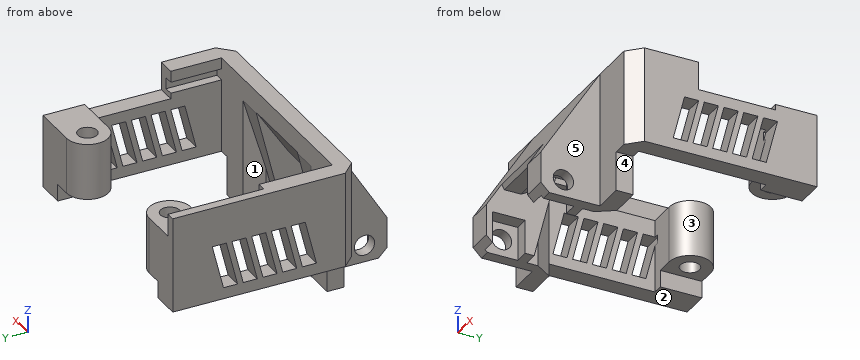
from build123d import *

# Parameters (mm, degrees)
SKETCH_1_W           = 44
SKETCH_1_H           = 34
EXTRUDE_1_DEPTH      = 24
CUT_EXTRUDE_1_DEPTH  = 31
SKETCH_5_W           = 23
SKETCH_5_H           = 10.5
EXTRUDE_4_DEPTH      = 1
EXTRUDE_5_DEPTH      = 23
SKETCH_7_R           = 1.8
CUT_EXTRUDE_2_DEPTH  = 23
CUT_EXTRUDE_4_DEPTH  = 19
CHAMFER_2_SIZE       = 2
CHAMFER_2_SIZE2      = 3
SKETCH_11_R          = 1.7
EXTRUDE_6_DEPTH      = 20
CUT_EXTRUDE_7_DEPTH  = 4
CHAMFER_3_SIZE       = 2.4
SKETCH_14_W          = 40.8
SKETCH_14_H          = 4
CUT_EXTRUDE_8_DEPTH  = 18
SKETCH_15_W          = 44
SKETCH_15_H          = 1
CUT_EXTRUDE_9_DEPTH  = 24
SKETCH_16_W          = 3.2
SKETCH_16_H          = 13.6
CUT_EXTRUDE_10_DEPTH = 5
SKETCH_17_W          = 1.6
SKETCH_17_H          = 4
CUT_EXTRUDE_11_DEPTH = 7.4
CUT_EXTRUDE_12_DEPTH = 7
SKETCH_19_W          = 1
SKETCH_19_H          = 10.5
CUT_EXTRUDE_13_DEPTH = 23
CHAMFER_4_SIZE       = 1.5
CHAMFER_5_SIZE       = 3
CHAMFER_5_SIZE2      = 2
CUT_EXTRUDE_START    = -3
SKETCH_20_W          = 14
SKETCH_20_H          = 11.956557484
CUT_EXTRUDE_14_DEPTH = 17
CHAMFER_6_SIZE       = 10
CHAMFER_6_SIZE_2     = 4
CHAMFER_7_SIZE       = 1
SKETCH_22_W          = 6.7
SKETCH_22_H          = 10
CUT_EXTRUDE_15_DEPTH = 10
SKETCH_24_W          = 6
SKETCH_24_H          = 5.8
CUT_EXTRUDE_16_DEPTH = 2.5


with BuildPart() as part:
    # Sketch 1 → Extrude 1 (new body)
    with BuildSketch(Plane.XY):
        with Locations((0, 27)):
            Rectangle(SKETCH_1_W, SKETCH_1_H)
    extrude(amount=EXTRUDE_1_DEPTH)

    # Sketch 2 → Cut-Extrude 1 (cut)
    with BuildSketch(Plane(origin=(0, 44, 0), x_dir=(1, 0, 0), z_dir=(0, 1, 0))):
        Polygon((-18.8, 0), (18.8, 0), (18.8, -20), (20.4, -20), (20.4, -22), (18.8, -22), (18.8, -24), (-18.8, -24), (-18.8, -22), (-20.4, -22), (-20.4, -20), (-18.8, -20), align=None)
    extrude(amount=-CUT_EXTRUDE_1_DEPTH, mode=Mode.SUBTRACT)



with BuildPart() as body_2:
    # Sketch 5 → Extrude 4 (new body)
    with BuildSketch(Plane(origin=(0, 0, 0), x_dir=(-1, 0, 0), z_dir=(0, 0, -1))):
        with Locations((0, 4.75)):
            Rectangle(SKETCH_5_W, SKETCH_5_H)
    extrude(amount=EXTRUDE_4_DEPTH)


with BuildPart() as part_1:
    add(part.part)

    add(body_2.part)  # Extrude 5 merges body 2
    # Sketch 6 → Extrude 5 (add)
    with BuildSketch(Plane(origin=(11.5, 0, 0), x_dir=(0, 0, -1), z_dir=(1, 0, 0))):
        Polygon((0, -0.5), (-7, -0.5), (-24, 10), (0, 10), align=None)
    extrude(amount=-EXTRUDE_5_DEPTH)

    # Sketch 7 → Cut-Extrude 2 (cut)
    with BuildSketch(Plane.ZY.offset(11.5)):
        with Locations(Location((3, 3.5, 0), (0, 0, 270))):
            Circle(SKETCH_7_R)
    extrude(amount=-CUT_EXTRUDE_2_DEPTH, mode=Mode.SUBTRACT)

    # Sketch 8 → Cut-Extrude 4 (cut)
    with BuildSketch(Plane.ZY.offset(9.5)):
        Polygon((0, 8), (20, 13), (0, 13), align=None)
    extrude(amount=-CUT_EXTRUDE_4_DEPTH, mode=Mode.SUBTRACT)

    # Chamfer 2
    chamfer_2_edges = [part_1.edges().sort_by_distance(p)[0] for p in [
        (9.5, 13, 10),
    ]]
    chamfer_2_side = [part_1.faces().sort_by_distance(p)[0] for p in [
        (-18.32664601, 13, 10),
    ]]
    chamfer(chamfer_2_edges, length=CHAMFER_2_SIZE, length2=CHAMFER_2_SIZE2, reference=chamfer_2_side[0])

    # Sketch 11 → Extrude 6 (add)
    # profile 1 of 2: a face of its own
    with BuildSketch(Plane(origin=(0, 0, 0), x_dir=(-1, 0, 0), z_dir=(0, 0, -1))):
        with BuildLine():
            Line((-14, 43), (-18.8, 43))
            Line((-18.8, 43), (-18.8, 35.6))
            Line((-18.8, 35.6), (-14, 35.6))
            ThreePointArc((-14, 35.6), (-10.3, 39.3), (-14, 43))
        make_face()
        with Locations((-14, 39.3)):
            Circle(SKETCH_11_R, mode=Mode.SUBTRACT)
    # profile 2 of 2: a face of its own
    with BuildSketch(Plane(origin=(0, 0, 0), x_dir=(-1, 0, 0), z_dir=(0, 0, -1))):
        with BuildLine():
            Line((18.8, 35.6), (14, 35.6))
            ThreePointArc((14, 35.6), (10.3, 39.3), (14, 43))
            Line((14, 43), (18.8, 43))
            Line((18.8, 43), (18.8, 35.6))
        make_face()
        with Locations((14, 39.3)):
            Circle(SKETCH_11_R, mode=Mode.SUBTRACT)
    extrude(amount=-EXTRUDE_6_DEPTH)

    # Sketch 13 → Cut-Extrude 7 (cut)
    with BuildSketch(Plane.ZY.offset(22)):
        Polygon((9, 34), (17, 36), (17, 33.5), (9, 31.5), align=None)
        Polygon((9, 30.5), (17, 32.5), (17, 30), (9, 28), align=None)
        Polygon((9, 27), (17, 29), (17, 26.5), (9, 24.5), align=None)
        Polygon((9, 23.5), (17, 25.5), (17, 23), (9, 21), align=None)
        Polygon((9, 20), (17, 22), (17, 19.5), (9, 17.5), align=None)
    cut_extrude_7 = extrude(amount=-CUT_EXTRUDE_7_DEPTH, mode=Mode.SUBTRACT)

    # Mirror 1: Cut-Extrude 7 across plane
    add(cut_extrude_7.mirror(Plane(origin=(0, 0, 0), x_dir=(0, 0, 1), z_dir=(1, 0, 0))), mode=Mode.SUBTRACT)

    # Chamfer 3
    chamfer_3_edges = [part_1.edges().sort_by_distance(p)[0] for p in [
        (22, 10, 12),
        (-22, 10, 12),
    ]]
    chamfer(chamfer_3_edges, length=CHAMFER_3_SIZE)

    # Sketch 14 → Cut-Extrude 8 (cut)
    with BuildSketch(Plane(origin=(0, 44, 0), x_dir=(1, 0, 0), z_dir=(0, 1, 0))):
        with Locations((0, -22)):
            Rectangle(SKETCH_14_W, SKETCH_14_H)
    extrude(amount=-CUT_EXTRUDE_8_DEPTH, mode=Mode.SUBTRACT)

    # Sketch 15 → Cut-Extrude 9 (cut)
    with BuildSketch(Plane(origin=(0, 0, 0), x_dir=(-1, 0, 0), z_dir=(0, 0, -1))):
        with Locations((0, 43.5)):
            Rectangle(SKETCH_15_W, SKETCH_15_H)
    extrude(amount=-CUT_EXTRUDE_9_DEPTH, mode=Mode.SUBTRACT)

    # Sketch 16 → Cut-Extrude 10 (cut)
    with BuildSketch(Plane.XY.offset(24)):
        with Locations((20.4, 28.8)):
            Rectangle(SKETCH_16_W, SKETCH_16_H)
    extrude(amount=-CUT_EXTRUDE_10_DEPTH, mode=Mode.SUBTRACT)

    # Sketch 17 → Cut-Extrude 11 (cut)
    with BuildSketch(Plane(origin=(0, 43, 0), x_dir=(1, 0, 0), z_dir=(0, 1, 0))):
        with Locations((21.2, -22)):
            Rectangle(SKETCH_17_W, SKETCH_17_H)
    extrude(amount=-CUT_EXTRUDE_11_DEPTH, mode=Mode.SUBTRACT)

    # Sketch 18 → Cut-Extrude 12 (cut)
    with BuildSketch(Plane(origin=(0, 0, 0), x_dir=(-1, 0, 0), z_dir=(0, 0, -1))):
        Polygon((-22, 43), (-17, 43), (-17, 10), (-19.6, 10), (-22, 12.4), align=None)
        Polygon((22, 12.4), (19.6, 10), (17, 10), (17, 43), (22, 43), align=None)
    extrude(amount=-CUT_EXTRUDE_12_DEPTH, mode=Mode.SUBTRACT)

    # Sketch 19 → Cut-Extrude 13 (cut)
    with BuildSketch(Plane.ZY.offset(11.5)):
        with Locations((-0.5, 4.75)):
            Rectangle(SKETCH_19_W, SKETCH_19_H)
    extrude(amount=-CUT_EXTRUDE_13_DEPTH, mode=Mode.SUBTRACT)

    # Chamfer 4
    chamfer_4_edges = [part_1.edges().sort_by_distance(p)[0] for p in [
        (0, -0.5, 0),
    ]]
    chamfer(chamfer_4_edges, length=CHAMFER_4_SIZE)

    # Chamfer 5
    chamfer_5_edges = [part_1.edges().sort_by_distance(p)[0] for p in [
        (-9.5, 13, 10),
    ]]
    chamfer_5_side = [part_1.faces().sort_by_distance(p)[0] for p in [
        (-9.5, 11.333333333, 6.666666667),
    ]]
    chamfer(chamfer_5_edges, length=CHAMFER_5_SIZE, length2=CHAMFER_5_SIZE2, reference=chamfer_5_side[0])

    # Sketch 20 → Cut-Extrude 14 (cut)
    with BuildSketch(Plane(origin=(0, 0, 0), x_dir=(1, 0, 0), z_dir=(0, 1, 0)).offset(CUT_EXTRUDE_START)):
        with Locations((0, -4.591721258)):
            Rectangle(SKETCH_20_W, SKETCH_20_H)
    extrude(amount=CUT_EXTRUDE_14_DEPTH, mode=Mode.SUBTRACT)

    # Chamfer 6
    # the kernel refuses this chamfer: 10, 4 mm, written as the material it takes off along each edge
    with BuildSketch(Plane(origin=(7, 10.6425, 10.57), x_dir=(0, 0.254985552304956, 0.966944863017399), z_dir=(-1, 0, 0))) as chamfer_6_piece_1:
        Polygon((CHAMFER_6_SIZE * 0.999917387214, -CHAMFER_6_SIZE * 0.0128537444865), (-CHAMFER_6_SIZE_2 * 0.254985552305, -CHAMFER_6_SIZE_2 * 0.966944863017), (0, 0), align=None)
    extrude(amount=14, mode=Mode.SUBTRACT)

    # Chamfer 7
    chamfer_7_edges = [part_1.edges().sort_by_distance(p)[0] for p in [
        (0, 1.705, 10.57),
        (0, 6.6425, 10.57),
    ]]
    chamfer(chamfer_7_edges, length=CHAMFER_7_SIZE)

    # Sketch 22 → Cut-Extrude 15 (cut)
    with BuildSketch(Plane(origin=(0, 43, 0), x_dir=(1, 0, 0), z_dir=(0, 1, 0))):
        with Locations((13.65, -5)):
            Rectangle(SKETCH_22_W, SKETCH_22_H)
        with Locations((-13.65, -5)):
            Rectangle(SKETCH_22_W, SKETCH_22_H)
    extrude(amount=-CUT_EXTRUDE_15_DEPTH, mode=Mode.SUBTRACT)

    # Sketch 24 → Cut-Extrude 16 (cut)
    with BuildSketch(Plane(origin=(-7, 0, 0), x_dir=(0, 0, -1), z_dir=(1, 0, 0))):
        with Locations((-3, 3.5)):
            Rectangle(SKETCH_24_W, SKETCH_24_H)
    cut_extrude_16 = extrude(amount=-CUT_EXTRUDE_16_DEPTH, mode=Mode.SUBTRACT)

    # Mirror 2: Cut-Extrude 16 across plane
    add(cut_extrude_16.mirror(Plane(origin=(0, 0, 0), x_dir=(0, 0, 1), z_dir=(1, 0, 0))), mode=Mode.SUBTRACT)


solid = part_1.part
Design review of the part built by this model. Coordinates are the model's own, in mm. Face numbers are marked on the shaded views. A direction names the side the tool comes from. Give positions to 0.01 mm unless a question says otherwise; leave off trailing zeros. Write each loop counter-clockwise with the first axis right and the second up, starting at its lowest first coordinate (ties: lowest second). Pieces come first, ordered by that corner, then holes. Notation, with made-up numbers: M 62,61 L 95,61 A25 cw 95,81 Z; hole C 87,-1 d8. An arc over 180 degrees is marked long. Answer as a JSON object with one key per item and string values. Group by question number.
1) We need section D-D (x = -4). Give the boundary of the cut face in (y, z) (1 decimal), and give its area (3 significant figures).
2) We need section B-B (z = 3). Count the separate pieces of the cut face and the enclosed holes in it, and give its area (4 significant figures).
3) Clearance check with flat-ended pins moving along their axes: pin 1 Ø0.8 at (x, y) = (-21, 21) entering from -Z; pin 2 Ø4 at (x, z) = (-15.5, 13.5) entering from -Y; pin 3 Ø2 at (x, y) = (11, 37) entering from -Z. State where each tip first meets the part, or that it passes through.
4) We need section A-A (y = 14.5). Give the boundary of the cut face in (x, z), and give its area (3 significant figures).
5) We need section C-C (y = 39.3). Give the boundary of the cut face in (x, z).
6) For line 1 along Y through (x, z) = (-14, 17.75); line 2 along X through (y, z) = (39, 9.25); line 3 along X through (y, z) = (9.5, 5.5), list the stretches that pass through material, from the lowest coordinate up.
7) Tool access review of the marked faces 1, 2, 3, 4 and 5: name each direction out of +Z, -Z, +X, -X, +Y, -Y from which nothing blocks a thin tool from reaching the whole face with its end or side.
Answer key:
{
 "1": {"outline": "M 2.2,11.4 L 2.7,10.6 L 5.6,10.6 L 7.2,11.4 L 13,20.2 L 13,24 L 10,24 Z", "area": "64.6 mm²"},
 "2": {"separate pieces": "4", "enclosed holes": "0", "area": "83.85 mm²"},
 "3": {"pin 1": "stops at z = 7", "pin 2": "stops at y = 10", "pin 3": "stops at z = 10"},
 "4": {"outline": "M -22,7 L -18.8,7 L -18.8,20 L -20.4,20 L -20.4,22 L -18.8,22 L -18.8,24 L -22,24 Z; M 18.8,7 L 22,7 L 22,24 L 18.8,24 L 18.8,22 L 20.4,22 L 20.4,20 L 18.8,20 Z", "area": "102 mm²"},
 "5": {"outline": "M -22,7 L -17,7 L -17,10 L -15.7,10 L -15.7,20 L -20.4,20 L -20.4,24 L -22,24 Z; M -12.3,10 L -10.3,10 L -10.3,20 L -12.3,20 Z; M 10.3,10 L 12.3,10 L 12.3,20 L 10.3,20 Z; M 15.7,10 L 17,10 L 17,7 L 22,7 L 22,20 L 15.7,20 Z"},
 "6": {"line 1": "y = 10 to 13, 35.6 to 37.6, 41 to 43", "line 2": "x = -22 to -17, 17 to 22", "line 3": "x = -11.5 to -9.5, 9.5 to 11.5"},
 "7": {"face 1": "-Z", "face 2": "-Z, -X, +Y, -Y", "face 3": "+Z, -Z", "face 4": "-Z, +X, +Y, -Y", "face 5": "+Z, -Z, +X, -Y"}
}
